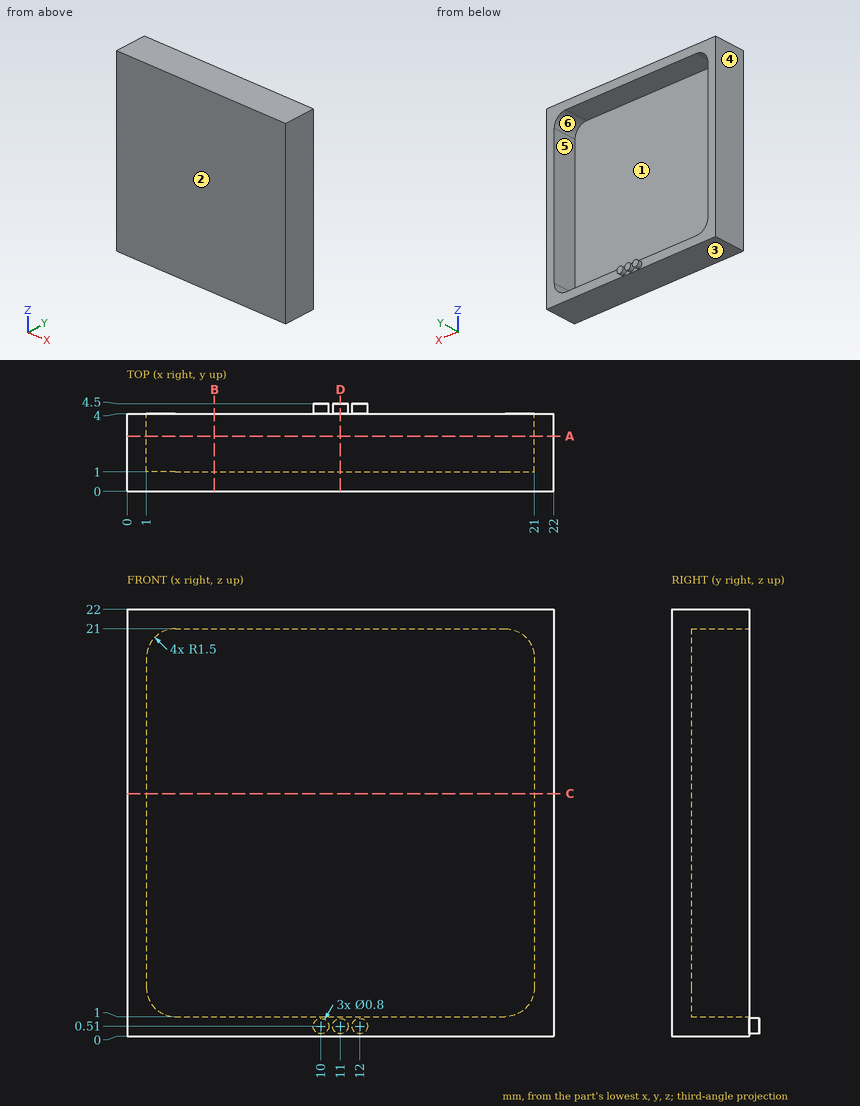
Geometry: see drawing. Coordinates: mm, zero at the bounding-box minimum. A direction names the side the tool comes from. Coordinates: 2 decimals unless noted, no trailing zeros. Loops run counter-clockwise (first coordinate to the right, second up) from the corner with the lowest first, then second, coordinate; pieces in that order, holes last. Notation, with made-up numbers: (0.25, 38) - (26.25, 38) arc R20 ccw to (26.25, 77) - close; hole circle Ø5 at (58.5, -35). An arc over 180 degrees is marked (long way). Return JSON: item names as keys, results as strings.
Q1. Section B-B, the plane x = 4.5. Return loops of the section in (y, z), plus the area to 3 significant figures.
Results:
{"outline": "(0, 0) - (4, 0) - (4, 1) - (1, 1) - (1, 21) - (4, 21) - (4, 22) - (0, 22) - close", "area": "28.0 mm2"}
Q2. Section D-D, the plane x = 11. Return loops of the section in (y, z), plus the area to 3 significant figures.
Results:
{"outline": "(0, 0) - (4, 0) - (4, 0.11) - (4.5, 0.11) - (4.5, 0.91) - (4, 0.91) - (4, 1) - (1, 1) - (1, 21) - (4, 21) - (4, 22) - (0, 22) - close", "area": "28.4 mm2"}
Q3. Section C-C, the plane z = 12.5. Return loops of the section in (x, y), plus the area to 3 significant figures.
Results:
{"outline": "(0, 0) - (22, 0) - (22, 4) - (21, 4) - (21, 1) - (1, 1) - (1, 4) - (0, 4) - close", "area": "28.0 mm2"}
Q4. Section A-A, the plane y = 2.85. Return loops of the section in (x, z).
Results:
{"outline": "(0, 0) - (22, 0) - (22, 22) - (0, 22) - close; hole (1, 2.5) arc R1.5 ccw to (2.5, 1) - (19.5, 1) arc R1.5 ccw to (21, 2.5) - (21, 19.5) arc R1.5 ccw to (19.5, 21) - (2.5, 21) arc R1.5 ccw to (1, 19.5) - close"}
Q5. Access query for the marked faces 1 and 2. Directions: +Z, -Z, +X, -X, +Y, -Y. A direction counts if a zero-diameter tool reaches every point of the face in a straight line with its end or side. Return the directions, or none.
Results:
{"face 1": "+Y", "face 2": "+Z, -Z, +X, -X, -Y"}
Q6. Contact query for a flat-ended pin moving along its axis: P1, Ø6, axis at x = 17.5, z = 17, coming from the +Y side. Output: stop coordinate, or through.
Results:
{"P1": "y = 1"}
Q7. Material intervals for line 1 along X through (y, z) = (1.8, 6.5); line 2 along Y through (x, z) = (2, 5.75), sorted ascending.
Results:
{"line 1": "0 to 1, 21 to 22", "line 2": "0 to 1"}
Q8. Mould query, pull axis Z, two halves, no side actions, for the marked faces 3, 4, 5 and 6. Classes: released by +Z, released by -Z, zero draft, split by the parting line, or undercut.
Results:
{"face 3": "released by -Z", "face 4": "zero draft", "face 5": "undercut", "face 6": "undercut"}
